Drawing for the job (mm, zero at the part's lowest x, y, z). A direction names the side the tool comes from. Give positions to 0.01 mm unless a question says otherwise; leave off trailing zeros. Loops run counter-clockwise (first coordinate to the right, second up) from the corner with the lowest first, then second, coordinate; pieces in that order, holes last. Notation, with made-up numbers: (22.25, 73.25) -> (74.25, 73.25) arc R19 cw to (74.25, 79.25) -> close; hole circle Ø6 at (22, 25). An arc over 180 degrees is marked (long way). Use CSV: the item, a comma, the result in double quotes. Start each with the question number.
(1) Pull direction Z, two halves, no side cores. Call the marked faces 1, 2 and 3: pulls with the +Z half, pulls with the -Z half, needs draft (parallel to the pull), parting line crosses it, or undercut.
(2) Cut at D-D on x = 12.5. Write the cut outline in (y, z).
(3) 3-axis set-ups, long thin cutter, end or side, ignore diameter. For the marked faces 4, 5 and 6: which of +Z, -Z, +X, -X, +Y, -Y reach the whole face in a straight line?
(4) Cut at C-C on y = 17. Write the cut outline in (x, z), then the cut area to 3 significant figures.
(5) Drill centre lines: probe 1 along Y at (x, z) = (32, 1); probe 2 along X at (y, z) = (21.5, 28); probe 3 along X at (y, z) = (10, 28) (3 decimals). Where is each one in solid material? Low to high.
(6) Flat gauge pins, fed straight in: pin 1 (5 mm diameter, centred on x = 13, y = 17.5, fed in from +Z); pin 2 (3.5 mm diameter, centred on x = 32.1, y = 15, fed in from +Z). Where does each tip first touch, or does it go through?
(7) Cut at B-B on x = 32.1. Write the cut outline in (y, z).
(8) Cut at A-A on z = 21. Write the cut outline in (x, y), then the cut area to 3 significant figures.
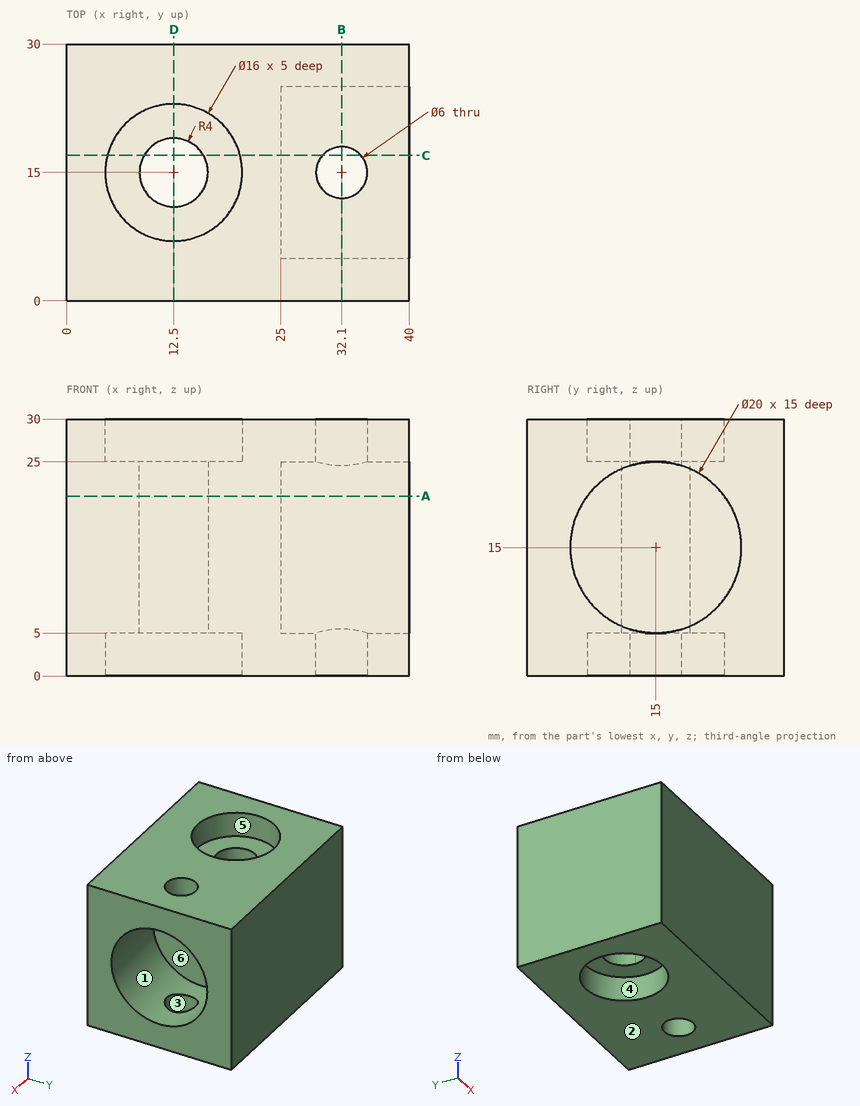
Check result:
1,face 1,"undercut"
1,face 2,"pulls with the -Z half"
1,face 3,"needs draft"
2,outline,"(0, 0) -> (7, 0) -> (7, 5) -> (11, 5) -> (11, 25) -> (7, 25) -> (7, 30) -> (0, 30) -> close; (19, 5) -> (23, 5) -> (23, 0) -> (30, 0) -> (30, 30) -> (23, 30) -> (23, 25) -> (19, 25) -> close"
3,face 4,"-Z"
3,face 5,"+Z"
3,face 6,"+X"
4,outline,"(0, 0) -> (4.75, 0) -> (4.75, 5) -> (9.04, 5) -> (9.04, 25) -> (4.75, 25) -> (4.75, 30) -> (0, 30) -> close; (15.96, 5) -> (20.25, 5) -> (20.25, 0) -> (29.86, 0) -> (29.86, 5.2) -> (25, 5.2) -> (25, 24.8) -> (29.86, 24.8) -> (29.86, 30) -> (20.25, 30) -> (20.25, 25) -> (15.96, 25) -> close; (34.34, 0) -> (40, 0) -> (40, 5.2) -> (34.34, 5.2) -> close; (34.34, 24.8) -> (40, 24.8) -> (40, 30) -> (34.34, 30) -> close"
4,area,"566 mm²"
5,probe 1,"0 to 12, 18 to 30"
5,probe 2,"0 to 7.84, 17.16 to 40"
5,probe 3,"0 to 6.255, 18.745 to 40"
6,pin 1,"z = 25"
6,pin 2,"through"
7,outline,"(0, 0) -> (12, 0) -> (12, 5.46) arc R10 cw to (12, 24.54) -> (12, 30) -> (0, 30) -> close; (18, 0) -> (30, 0) -> (30, 30) -> (18, 30) -> (18, 24.54) arc R10 cw to (18, 5.46) -> close"
8,outline,"(0, 0) -> (40, 0) -> (40, 7) -> (25, 7) -> (25, 23) -> (40, 23) -> (40, 30) -> (0, 30) -> close; hole circle Ø8 at (12.5, 15)"
8,area,"910 mm²"
